Model file for the job. Use its own axes, mm. Face numbers are marked on the shaded views. A direction names the side the tool comes from. Round coordinates to 2 decimals unless told otherwise and drop trailing zeros. Loops run counter-clockwise (first coordinate to the right, second up) from the corner with the lowest first, then second, coordinate; pieces in that order, holes last. Notation, with made-up numbers: (53.25, 6.25) -> (81.25, 6.25) arc R31 ccw to (81.25, 37.25) -> close; hole circle Ø10 at (-31.5, 54). An arc over 180 degrees is marked (long way). Use a Markdown table: item, result.
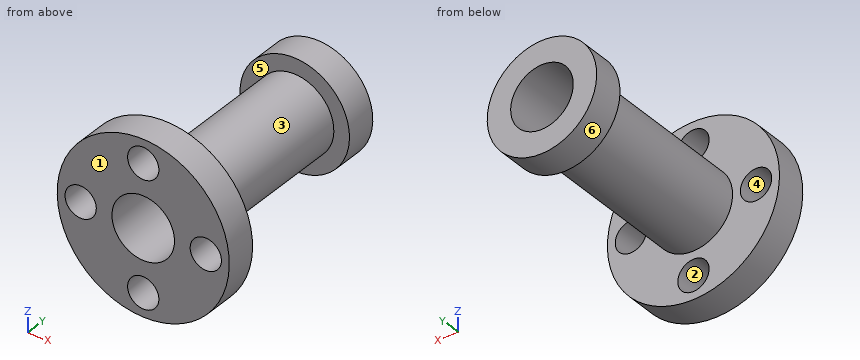
from build123d import *

# Parameters (mm, degrees)
SKETCH_2_R          = 4
CUT_EXTRUDE_1_DEPTH = 31.6
SKETCH_4_R          = 2
CUT_EXTRUDE_2_DEPTH = 31.6


with BuildPart() as part:
    # Эскиз1 → Повернуть1 (revolve)
    with BuildSketch(Plane.XY, mode=Mode.PRIVATE) as revolve_1_sk:
        Polygon((0, 0), (0, 30), (7, 30), (7, 26), (5, 26), (5, 4), (11, 4), (11, 0), align=None)
    revolve(revolve_1_sk.sketch.rotate(Axis((0, 0, 0), (0, 1, 0)), 90), axis=Axis((0, 0, 0), (0, 1, 0)))

    # Эскиз2 → Вырез-Вытянуть1 (cut)
    with BuildSketch(Plane(origin=(0, 30, 0), x_dir=(1, 0, 0), z_dir=(0, 1, 0))):
        with Locations(Location((0, 0, 0), (0, 0, 270))):
            Circle(SKETCH_2_R)
    extrude(amount=-CUT_EXTRUDE_1_DEPTH, mode=Mode.SUBTRACT)

    # Эскиз4 → Вырез-Вытянуть2 (cut)
    with BuildSketch(Plane(origin=(0, 4, 0), x_dir=(1, 0, 0), z_dir=(0, 1, 0))):
        with Locations(Location((8, 0, 0), (0, 0, 270))):
            Circle(SKETCH_4_R)
        with Locations(Location((0, 8, 0), (0, 0, 270))):
            Circle(SKETCH_4_R)
        with Locations(Location((-8, 0, 0), (0, 0, 270))):
            Circle(SKETCH_4_R)
        with Locations(Location((0, -8, 0), (0, 0, 270))):
            Circle(SKETCH_4_R)
    extrude(amount=-CUT_EXTRUDE_2_DEPTH, mode=Mode.SUBTRACT)


solid = part.part
Q1. Pull direction X, two halves, no side cores. Call the marked faces 1, 2 and 3: released by +X, released by -X, zero draft, split by the parting line, or undercut.
Results list:
| item | result |
|---|---|
| face 1 | zero draft |
| face 2 | undercut |
| face 3 | split by the parting line |
Q2. Band-saw the part on C-C, the plane y = 2.25. Give the cut face in (x, z), plus the area to 3 significant figures.
Results list:
| item | result |
|---|---|
| outline | circle Ø22 at (0, 0); hole circle Ø4 at (-8, 0); hole circle Ø8 at (0, 0); hole circle Ø4 at (0, -8); hole circle Ø4 at (0, 8); hole circle Ø4 at (8, 0) |
| area | 280 mm² |
Q3. Tool access for the marked faces 4, 5 and 6: list every direction of +Z, -Z, +X, -X, +Y, -Y with a clear straight run to the whole face (end or side of a thin tool).
Results list:
| item | result |
|---|---|
| face 4 | -Y |
| face 5 | none |
| face 6 | +Y |
Q4. Drill centre lines: L1, parallel to X at y = 2.1, z = 0; L2, parallel to Y at x = 5.75, z = 1.5; L3, parallel to X at y = 16.25, z = 0. Where is each one in solid material? Low to high. Write a range as from..to.
Results list:
| item | result |
|---|---|
| L1 | x = -11..-10, -6..-4, 4..6, 10..11 |
| L2 | y = 0..4, 26..30 |
| L3 | x = -5..-4, 4..5 |
Q5. Flat gauge pins, fed straight in: pin 1 (5 mm diameter, centred on y = 9, z = 1.5, fed in from +X); pin 2 (3.5 mm diameter, centred on x = 8, z = 0, fed in from -Y); pin 3 (6 mm diameter, centred on y = 8, z = -4, fed in from +X). Where does each tip first touch, or does it go through?
Results list:
| item | result |
|---|---|
| pin 1 | stops at x = 5 |
| pin 2 | stops at y = 26 |
| pin 3 | stops at x = 4.9 |
Q6. Band-saw the part on D-D, the plane x = -5.5. Give the cut face in (y, z), plus the area to 3 significant figures.
Results list:
| item | result |
|---|---|
| outline | (0, -9.53) -> (4, -9.53) -> (4, 9.53) -> (0, 9.53) -> close; (26, -4.33) -> (30, -4.33) -> (30, 4.33) -> (26, 4.33) -> close |
| area | 111 mm² |
Q7. Band-saw the part on B-B, the plane z = 0. Give the cut face in (x, y), plus the area to 3 significant figures.
Results list:
| item | result |
|---|---|
| outline | (-11, 0) -> (-10, 0) -> (-10, 4) -> (-11, 4) -> close; (-7, 26) -> (-5, 26) -> (-5, 4) -> (-6, 4) -> (-6, 0) -> (-4, 0) -> (-4, 30) -> (-7, 30) -> close; (4, 0) -> (6, 0) -> (6, 4) -> (5, 4) -> (5, 26) -> (7, 26) -> (7, 30) -> (4, 30) -> close; (10, 0) -> (11, 0) -> (11, 4) -> (10, 4) -> close |
| area | 92.0 mm² |
Q8. Band-saw the part on A-A, the plane x = 0. Give the cut face in (y, z), plus the area to 3 significant figures.
Results list:
| item | result |
|---|---|
| outline | (0, -11) -> (4, -11) -> (4, -10) -> (0, -10) -> close; (0, -6) -> (4, -6) -> (4, -5) -> (26, -5) -> (26, -7) -> (30, -7) -> (30, -4) -> (0, -4) -> close; (0, 4) -> (30, 4) -> (30, 7) -> (26, 7) -> (26, 5) -> (4, 5) -> (4, 6) -> (0, 6) -> close; (0, 10) -> (4, 10) -> (4, 11) -> (0, 11) -> close |
| area | 92.0 mm² |
